```python
from build123d import *

# Parameters (mm, degrees)
SKETCH1_W           = 138
SKETCH1_H           = 32
BOSS_EXTRUDE1_DEPTH = 42
SKETCH2_R           = 2
BOSS_EXTRUDE2_DEPTH = 5
FILLET1_R           = 6
FILLET2_R           = 3


with BuildPart() as part:
    # Sketch1 → Boss-Extrude1 (new body)
    with BuildSketch(Plane(origin=(0, 0, 0), x_dir=(1, 0, 0), z_dir=(0, 1, 0))):
        with Locations((69, 16)):
            Rectangle(SKETCH1_W, SKETCH1_H)
    extrude(amount=BOSS_EXTRUDE1_DEPTH)

    # Sketch2 → Boss-Extrude2 (add)
    with BuildSketch(Plane.ZY):
        with Locations(Location((-12, 40, 0), (0, 0, 90))):
            Circle(SKETCH2_R)
        with Locations(Location((-20, 40, 0), (0, 0, 90))):
            Circle(SKETCH2_R)
    extrude(amount=BOSS_EXTRUDE2_DEPTH)

    # Fillet1
    fillet1_edges = [part.edges().sort_by_distance(p)[0] for p in [
        (0, 21, -32),
        (0, 21, 0),
    ]]
    fillet(fillet1_edges, radius=FILLET1_R)

    # Fillet2
    # the kernel refuses this fillet: 3 mm, written as the material it takes off along each edge
    with BuildSketch(Plane(origin=(135, 39, -3), x_dir=(1, 0, 0), z_dir=(0, 0, 1))) as fillet2_piece_1_section:
        Polygon((0, 0), (FILLET2_R * 1.02, 0), (FILLET2_R * 1.02, FILLET2_R * 1.02), (0, FILLET2_R * 1.02), align=None)
    fillet2_piece_1 = extrude(amount=FILLET2_R * 1.02, mode=Mode.PRIVATE)
    fillet2_piece_1 = fillet2_piece_1 - Plane(origin=(135, 39, -3), x_dir=(-0.7071067811865475, -0.7071067811865475, 0), z_dir=(0, 0, 1)) * Sphere(FILLET2_R, mode=Mode.PRIVATE)
    add(fillet2_piece_1, mode=Mode.SUBTRACT)
    with BuildSketch(Plane(origin=(135, 39, -29), x_dir=(0, 1, 0), z_dir=(1, 0, 0))) as fillet2_piece_2_section:
        Polygon((0, 0), (FILLET2_R * 1.02, 0), (FILLET2_R * 1.02, -FILLET2_R * 1.02), (0, -FILLET2_R * 1.02), align=None)
    fillet2_piece_2 = extrude(amount=FILLET2_R * 1.02, mode=Mode.PRIVATE)
    fillet2_piece_2 = fillet2_piece_2 - Plane(origin=(135, 39, -29), x_dir=(0, -0.7071067811865475, 0.7071067811865475), z_dir=(1, 0, 0)) * Sphere(FILLET2_R, mode=Mode.PRIVATE)
    add(fillet2_piece_2, mode=Mode.SUBTRACT)
    with BuildSketch(Plane(origin=(135, 3, -3), x_dir=(0, -1, 0), z_dir=(0, 0, 1))) as fillet2_piece_3_section:
        Polygon((0, 0), (FILLET2_R * 1.02, 0), (FILLET2_R * 1.02, FILLET2_R * 1.02), (0, FILLET2_R * 1.02), align=None)
    fillet2_piece_3 = extrude(amount=FILLET2_R * 1.02, mode=Mode.PRIVATE)
    fillet2_piece_3 = fillet2_piece_3 - Plane(origin=(135, 3, -3), x_dir=(-0.7071067811865475, 0.7071067811865475, 0), z_dir=(0, 0, 1)) * Sphere(FILLET2_R, mode=Mode.PRIVATE)
    add(fillet2_piece_3, mode=Mode.SUBTRACT)
    with BuildSketch(Plane(origin=(135, 3, -29), x_dir=(1, 0, 0), z_dir=(0, -1, 0))) as fillet2_piece_4_section:
        Polygon((0, 0), (FILLET2_R * 1.02, 0), (FILLET2_R * 1.02, -FILLET2_R * 1.02), (0, -FILLET2_R * 1.02), align=None)
    fillet2_piece_4 = extrude(amount=FILLET2_R * 1.02, mode=Mode.PRIVATE)
    fillet2_piece_4 = fillet2_piece_4 - Plane(origin=(135, 3, -29), x_dir=(-0.7071067811865475, 0, 0.7071067811865475), z_dir=(0, -1, 0)) * Sphere(FILLET2_R, mode=Mode.PRIVATE)
    add(fillet2_piece_4, mode=Mode.SUBTRACT)
    with BuildSketch(Plane(origin=(138, 42, -3), x_dir=(0, -1, 0), z_dir=(0, 0, -1)), Plane(origin=(138, 0, -3), x_dir=(-1, 0, 0), z_dir=(0, 0, -1))) as fillet2_piece_5:
        with BuildLine():
            CenterArc((FILLET2_R, FILLET2_R), FILLET2_R, 180, 90)
            Line((0, FILLET2_R), (0, 0))
            Line((0, 0), (FILLET2_R, 0))
        make_face()
    extrude(amount=26, mode=Mode.SUBTRACT)
    with BuildSketch(Plane(origin=(0, 42, -12), x_dir=(1, 0, 0), z_dir=(0, 0, 1))) as fillet2_piece_6_section:
        with BuildLine():
            CenterArc((FILLET2_R, -FILLET2_R), FILLET2_R, 90, 90)
            Line((0, -FILLET2_R), (0, 0))
            Line((0, 0), (FILLET2_R, 0))
        make_face()
    fillet2_piece_6 = extrude(amount=6, mode=Mode.PRIVATE)
    fillet2_piece_6 = fillet2_piece_6 - Plane(origin=(0.483529934, 40, -12), x_dir=(0, 1, 0), z_dir=(1, 0, 0)) * Cylinder(2, 24, mode=Mode.PRIVATE)
    add(fillet2_piece_6, mode=Mode.SUBTRACT)
    with BuildSketch(Plane(origin=(135, 42, -32), x_dir=(0, 0, 1), z_dir=(-1, 0, 0)), Plane(origin=(6, 0, 0), x_dir=(0, 1, 0), z_dir=(1, 0, 0))) as fillet2_piece_7:
        with BuildLine():
            CenterArc((FILLET2_R, -FILLET2_R), FILLET2_R, 90, 90)
            Line((0, -FILLET2_R), (0, 0))
            Line((0, 0), (FILLET2_R, 0))
        make_face()
    extrude(amount=129, mode=Mode.SUBTRACT)
    with BuildSketch(Plane(origin=(0, 42, -20), x_dir=(1, 0, 0), z_dir=(0, 0, 1))) as fillet2_piece_8_section:
        with BuildLine():
            CenterArc((FILLET2_R, -FILLET2_R), FILLET2_R, 90, 90)
            Line((0, -FILLET2_R), (0, 0))
            Line((0, 0), (FILLET2_R, 0))
        make_face()
    fillet2_piece_8 = extrude(amount=8, mode=Mode.PRIVATE)
    fillet2_piece_8 = fillet2_piece_8 - Plane(origin=(0.736023116, 40, -20), x_dir=(0, 1, 0), z_dir=(1, 0, 0)) * Cylinder(2, 28, mode=Mode.PRIVATE)
    fillet2_piece_8 = fillet2_piece_8 - Plane(origin=(0.736023116, 40, -12), x_dir=(0, 1, 0), z_dir=(1, 0, 0)) * Cylinder(2, 28, mode=Mode.PRIVATE)
    add(fillet2_piece_8, mode=Mode.SUBTRACT)
    with BuildSketch(Plane(origin=(0, 42, -26), x_dir=(1, 0, 0), z_dir=(0, 0, 1))) as fillet2_piece_9_section:
        with BuildLine():
            CenterArc((FILLET2_R, -FILLET2_R), FILLET2_R, 90, 90)
            Line((0, -FILLET2_R), (0, 0))
            Line((0, 0), (FILLET2_R, 0))
        make_face()
    fillet2_piece_9 = extrude(amount=6, mode=Mode.PRIVATE)
    fillet2_piece_9 = fillet2_piece_9 - Plane(origin=(0.914317851, 40, -20), x_dir=(0, 1, 0), z_dir=(1, 0, 0)) * Cylinder(2, 24, mode=Mode.PRIVATE)
    add(fillet2_piece_9, mode=Mode.SUBTRACT)
    with BuildSketch(Plane(origin=(0, 0, -26), x_dir=(1, 0, 0), z_dir=(0, 0, 1))) as fillet2_piece_10:
        with BuildLine():
            CenterArc((FILLET2_R, FILLET2_R), FILLET2_R, 180, 90)
            Line((0, FILLET2_R), (0, 0))
            Line((0, 0), (FILLET2_R, 0))
        make_face()
    extrude(amount=20, mode=Mode.SUBTRACT)
    with BuildSketch(Plane(origin=(6, 0, -6), x_dir=(0, 0, 1), z_dir=(1, 0, 0))) as fillet2_piece_11:
        with BuildLine():
            CenterArc((6 - FILLET2_R, -FILLET2_R), FILLET2_R, 0, 90)
            Line((6, -FILLET2_R), (6, 0))
            Line((6, 0), (6 - FILLET2_R, 0))
        make_face()
    revolve(axis=Axis((6, 0, -6), (0, -1, 0)), revolution_arc=90, mode=Mode.SUBTRACT)
    with BuildSketch(Plane(origin=(6, 0, -26), x_dir=(-1, 0, 0), z_dir=(0, 0, 1))) as fillet2_piece_12:
        with BuildLine():
            CenterArc((6 - FILLET2_R, -FILLET2_R), FILLET2_R, 0, 90)
            Line((6, -FILLET2_R), (6, 0))
            Line((6, 0), (6 - FILLET2_R, 0))
        make_face()
    revolve(axis=Axis((6, 0, -26), (0, -1, 0)), revolution_arc=90, mode=Mode.SUBTRACT)
    with BuildSketch(Plane(origin=(6, 42, 0), x_dir=(0, -1, 0), z_dir=(1, 0, 0)), Plane(origin=(135, 0, -32), x_dir=(0, 0, 1), z_dir=(-1, 0, 0))) as fillet2_piece_13:
        with BuildLine():
            CenterArc((FILLET2_R, FILLET2_R), FILLET2_R, 180, 90)
            Line((0, FILLET2_R), (0, 0))
            Line((0, 0), (FILLET2_R, 0))
        make_face()
    extrude(amount=129, mode=Mode.SUBTRACT)
    with BuildSketch(Plane(origin=(6, 42, -6), x_dir=(0, 0, 1), z_dir=(1, 0, 0))) as fillet2_piece_14:
        with BuildLine():
            CenterArc((6 - FILLET2_R, FILLET2_R), FILLET2_R, 270, 90)
            Line((6 - FILLET2_R, 0), (6, 0))
            Line((6, 0), (6, FILLET2_R))
        make_face()
    revolve(axis=Axis((6, 42, -6), (0, -1, 0)), revolution_arc=90, mode=Mode.SUBTRACT)
    with BuildSketch(Plane(origin=(6, 42, -26), x_dir=(-1, 0, 0), z_dir=(0, 0, 1))) as fillet2_piece_15:
        with BuildLine():
            CenterArc((6 - FILLET2_R, FILLET2_R), FILLET2_R, 270, 90)
            Line((6, FILLET2_R), (6, 0))
            Line((6, 0), (6 - FILLET2_R, 0))
        make_face()
    revolve(axis=Axis((6, 42, -26), (0, -1, 0)), revolution_arc=90, mode=Mode.SUBTRACT)
    with BuildSketch(Plane(origin=(138, 3, -32), x_dir=(0, 0, 1), z_dir=(0, 1, 0)), Plane(origin=(138, 3, 0), x_dir=(-1, 0, 0), z_dir=(0, 1, 0))) as fillet2_piece_16:
        with BuildLine():
            CenterArc((FILLET2_R, -FILLET2_R), FILLET2_R, 90, 90)
            Line((0, -FILLET2_R), (0, 0))
            Line((0, 0), (FILLET2_R, 0))
        make_face()
    extrude(amount=36, mode=Mode.SUBTRACT)


solid = part.part
```
For this review, take the finished solid that the model builds, in its own axes (mm). Round coordinates to 2 decimals unless told otherwise and drop trailing zeros. Order: outer loops, then holes, each group sorted by start corner. A loop starts at its lowest first (then second) coordinate and runs counter-clockwise, first axis right, second up.
Q1. We need section A-A, the plane z = -16.5. Give the boundary of the cut face in (x, y), plus the area to 3 significant figures.
Findings below:
outline: (0, 3) arc R3 ccw to (3, 0) - (135, 0) arc R3 ccw to (138, 3) - (138, 39) arc R3 ccw to (135, 42) - (3, 42) arc R3 ccw to (0, 39) - close
area: 5,790 mm2
Q2. Wall thickness on line 1 (X direction, y = 3.5, z = -6.5); line 2 (X direction, y = 32.5, z = -1.5); line 3 (Y direction, x = 29.5, z = -1.5): over which ranges is each line inside the solid? List them lowest first.
Findings below:
line 1: x = 0 to 138
line 2: x = 2.03 to 137.6
line 3: y = 0.4 to 41.6
Q3. Mouldability with a two-part tool opening along Z and no side actions: class faces 1 (the flat face through (70, 21, -32)), 2 (the cylindrical face through (-1.833, 41.908, -20.601)), 3 (the cylindrical face through (-1.833, 41.908, -12.601)), 4 (the cylindrical face through (69.6, 41.14, -0.9)) as pulls with the +Z half, pulls with the -Z half, needs draft (parallel to the pull), parting line crosses it, or undercut.
Findings below:
face 1: pulls with the -Z half
face 2: undercut
face 3: undercut
face 4: pulls with the +Z half
Q4. We need section B-B, the plane y = 19.5. Give the boundary of the cut face in (x, z), plus the area to 3 significant figures.
Findings below:
outline: (0, -26) arc R6 ccw to (6, -32) - (135, -32) arc R3 ccw to (138, -29) - (138, -3) arc R3 ccw to (135, 0) - (6, 0) arc R6 ccw to (0, -6) - close
area: 4,400 mm2
Q5. Insertion check: P1, Ø10, axis at y = 29, z = -18.5, coming from the -X side. The pin has a flat end and moves straight along its axis. Give the tip position at first contact, or say it passes through.
Findings below:
P1: stops at x = 0
